Autodesk Inventor part; units mm, degrees
ref_plane "YZ Plane" through (0, 0, 0) normal (1, 0, 0) x (0, 1, 0)
ref_plane "XZ Plane" through (0, 0, 0) normal (0, 1, 0) x (-1, 0, 0)
ref_plane "XY Plane" through (0, 0, 0) normal (0, 0, 1) x (1, 0, 0)
sketch "Sketch1" plane through (0, 0, 0) normal (0, 1, 0) x (-1, 0, 0)
  line L0 (18, 15) -> (-18, 15)
  line L1 (-18, 15) -> (-18, -15)
  line L2 (-18, -15) -> (18, -15)
  line L3 (18, -15) -> (18, 15)
  point P0 (0, 0)
  point P1 (18, 0)
  point P2 (0, 15)
  dimension "d0" = 36
  dimension "d1" = 30
extrude "Extrusion1" add sketch "Sketch1" along normal blind 5
sketch "Sketch2" plane through (0, 5, 0) normal (0, 1, 0) x (1, 0, 0)
  line L0 (-18, -15) -> (18, -15)
  line L1 (-18, -15) -> (18, -15)
  line L2 (18, -15) -> (18, -10)
  line L3 (18, -10) -> (-18, -10)
  line L4 (-18, -10) -> (-18, -15)
  point P0 (0, 0)
  dimension "d4" = 5
extrude "Extrusion2" add sketch "Sketch2" along normal blind 25
sketch "Sketch3" plane through (0, 0, 0) normal (0, -1, 0) x (1, 0, 0)
  circle A0 centre (6, -5.5) radius 8.5
  line L0 (-18, 15) -> (18, 15)
  line L1 (18, 15) -> (18, -15)
  point P0 (0, 0)
  dimension "dGalvo" = 17
  dimension "d8" = 20.5
  dimension "d9" = 3.5
extrude "Extrusion3" add sketch "Sketch3" along normal blind 23
sketch "Sketch4" plane through (-18, 0, 15) normal (0, 0, 1) x (1, 0, 0)
  circle A0 centre (15.5, 19.5) radius 8.5
  line L0 (0, 30) -> (36, 30)
  line L1 (0, 0) -> (0, 30)
  point P0 (18, 0)
  dimension "d12" = 17
  dimension "d13" = 2
  dimension "d14" = 15.5
extrude "Extrusion4" add sketch "Sketch4" along normal blind 23
sketch "Sketch5" plane through (18, 5, 10) normal (0, 0, -1) x (-1, 0, 0)
  circle A0 centre (20.5, 14.5) radius 8.5
  point P0 (18, -5)
extrude "Extrusion5" add sketch "Sketch5" along normal blind 6.38
sketch "Sketch6" plane through (0, 5, 0) normal (0, 1, 0) x (1, 0, 0)
  circle A0 centre (6, 5.5) radius 8.5
  point P0 (0, 0)
extrude "Extrusion6" add sketch "Sketch6" along normal blind 6.38
sketch "Sketch7" plane through (6, 11.38, -5.5) normal (0, 1, 0) x (1, 0, 0)
  line L0 (-2.1213, -2.8284) -> (2.8284, 2.1213)
  line L1 (2.8284, 2.1213) -> (2.1213, 2.8284)
  line L2 (2.1213, 2.8284) -> (-2.8284, -2.1213)
  line L3 (-2.8284, -2.1213) -> (-2.1213, -2.8284)
  circle A0 centre (0, 0) radius 8.5
  point P0 (-6, -5.5)
  point P1 (-2.4749, -2.4749)
  point P2 (0.3536, -0.3536)
  dimension "lenMirror" = 7
  dimension "thicknessMirror" = 1
extrude "Extrusion7" add sketch "Sketch7" along normal blind 13 contours L3 L2 L1 L0
sketch "Sketch8" plane through (-2.5, 19.5, 3.62) normal (0, 0, -1) x (-1, 0, 0)
  circle A0 centre (0, 0) radius 8.5
  line L0 (2.1213, 2.8284) -> (-2.8284, -2.1213)
  line L1 (-2.8284, -2.1213) -> (-2.1213, -2.8284)
  line L2 (-2.1213, -2.8284) -> (2.8284, 2.1213)
  line L3 (2.8284, 2.1213) -> (2.1213, 2.8284)
  point P0 (-2.5, -19.5)
  point P1 (2.4749, 2.4749)
  point P2 (-0.3536, 0.3536)
  dimension "d25" = 7
  dimension "d26" = 1
extrude "Extrusion8" add sketch "Sketch8" along normal blind 13 contours L3 L2 L1 L0
equation "\"d12\" = dGalvo"
equation "\"d15\" = depthGalvo"
equation "\"d19\" = depthGalvoHead"
equation "\"d25\" = lenMirror"
equation "\"d26\" = thicknessMirror"
equation "\"d27\" = depthMirror"
properties part number "galvos"
Model file for the job. Use its own axes, mm. A direction names the side the tool comes from. Coordinates: 2 decimals unless noted, no trailing zeros. Order: outer loops, then holes, each group sorted by start corner. A loop starts at its lowest first (then second) coordinate and runs counter-clockwise, first axis right, second up. Notation, with made-up numbers: M -34.5,67.25 L 11.5,67.25 A17 ccw 11.5,76.25 Z; hole C -38,-4.75 d7. An arc over 180 degrees is marked long. Return JSON: item names as keys, results as strings.
1. Drill centre lines: probe 1 along Z at (x, y) = (3, 24); probe 2 along Y at (x, z) = (-11.5, -0.5); probe 3 along Y at (x, z) = (0, 12). Where is each one in solid material? Low to high.
Ans:
{"probe 1": "3.62 to 38", "probe 2": "0 to 5", "probe 3": "0 to 30"}
2. Tool access for faces 4 (the face through (4, 12, 10)), 5 (the face through (4.893, -11.339, -13.928)), 6 (the face through (5.681, 17.789, -5.888)), 7 (the face through (-2.5, 19.5, -9.38)): list every direction of +Z, -Z, +X, -X, +Y, -Y with a clear straight run to the whole face (end or side of a thin tool).
Ans:
{"face 4": "none", "face 5": "-Y", "face 6": "-Z, +Y", "face 7": "-Z, +X, -X, +Y"}
3. Pull direction Y, two halves, no side cores. Call faces 1 (the face through (-4, 5, -2)), 2 (the face through (6, 24.38, -5.5)), 3 (the face through (6, -23, -5)): +Y half, -Y half, draft (parallel to the pull), parting line (faces both ways), or undercut.
Ans:
{"face 1": "undercut", "face 2": "+Y half", "face 3": "-Y half"}
4. Saw through at A-A (y = 19.5). Give the cut face in (x, z).
Ans:
{"outline": "M -18,10 L -11,10 L -11,3.62 L -3.21,3.62 L -3.21,-9.38 L -1.79,-9.38 L -1.79,3.62 L 6,3.62 L 6,10 L 18,10 L 18,15 L 6,15 L 6,38 L -11,38 L -11,15 L -18,15 Z; M 3.17,-3.38 L 8.12,-8.33 L 8.83,-7.62 L 3.88,-2.67 Z"}
5. Flat gauge pins, fed straight in: pin 1 (12 mm diameter, centred on y = -8.5, z = 5.5, fed in from -X); pin 2 (3 mm diameter, centred on x = -2, y = 19, fed in from -Z); pin 3 (8.5 mm diameter, centred on x = 6.5, z = -5, fed in from +Y); pin 4 (2 mm diameter, centred on x = 8.5, z = 29.5, fed in from -Y). Where does each tip first touch, or does it go through?
Ans:
{"pin 1": "x = -0.87", "pin 2": "z = -9.38", "pin 3": "y = 24.38", "pin 4": "through"}
6. Saw through at D-D (z = 17). Give the cut face in (x, y).
Ans:
{"outline": "C -2.5,19.5 d17"}
7. Saw through at B-B (z = -5.5). Give the cut face in (x, y), and give its area (3 significant figures).
Ans:
{"outline": "M -18,0 L -2.5,0 L -2.5,-23 L 14.5,-23 L 14.5,0 L 18,0 L 18,5 L 14.5,5 L 14.5,11.38 L 6.71,11.38 L 6.71,24.38 L 5.29,24.38 L 5.29,11.38 L -2.5,11.38 L -2.5,5 L -18,5 Z; M -5.33,21.62 L -0.38,16.67 L 0.33,17.38 L -4.62,22.33 Z", "area": "705 mm^2"}
8. Saw through at C-C (x = -12.5). Give the cut face in (y, z).
Ans:
{"outline": "M 0,-15 L 5,-15 L 5,10 L 30,10 L 30,15 L 0,15 Z"}
